```python
from build123d import *

# Parameters (mm, degrees)
SALIENTE_EXTRUIR1_DEPTH = 60
CORTAR_EXTRUIR1_DEPTH   = 10


with BuildPart() as part:
    # Croquis1 → Saliente-Extruir1 (new body)
    with BuildSketch(Plane.XY):
        with BuildLine():
            Line((-71.508108108, 44.822972973), (-71.508108108, 45.822972973))
            Line((-71.508108108, 45.822972973), (-21.508108108, 45.822972973))
            Line((-21.508108108, 45.822972973), (-21.508108108, 44.822972973))
            ThreePointArc((-21.508108108, 44.822972973), (-20.008108108, 43.322972973), (-21.508108108, 41.822972973))
            Line((-21.508108108, 41.822972973), (-21.508108108, 40.822972973))
            Line((-21.508108108, 40.822972973), (-71.508108108, 40.822972973))
            Line((-71.508108108, 40.822972973), (-71.508108108, 41.822972973))
            ThreePointArc((-71.508108108, 41.822972973), (-73.008108108, 43.322972973), (-71.508108108, 44.822972973))
        make_face()
    extrude(amount=SALIENTE_EXTRUIR1_DEPTH)

    # Croquis3 → Cortar-Extruir1 (cut)
    with BuildSketch(Plane(origin=(0, 0, 0), x_dir=(-1, 0, 0), z_dir=(0, 0, -1))):
        with BuildLine():
            Line((36.508108108, 41.322972973), (36.508108108, 40.822972973))
            Line((36.508108108, 40.822972973), (56.508108108, 40.822972973))
            Line((56.508108108, 40.822972973), (56.508108108, 41.322972973))
            ThreePointArc((56.508108108, 41.322972973), (55.92232167, 42.737186535), (54.508108108, 43.322972973))
            Line((54.508108108, 43.322972973), (38.508108108, 43.322972973))
            ThreePointArc((38.508108108, 43.322972973), (37.093894546, 42.737186535), (36.508108108, 41.322972973))
        make_face()
    extrude(amount=-CORTAR_EXTRUIR1_DEPTH, mode=Mode.SUBTRACT)


solid = part.part
```
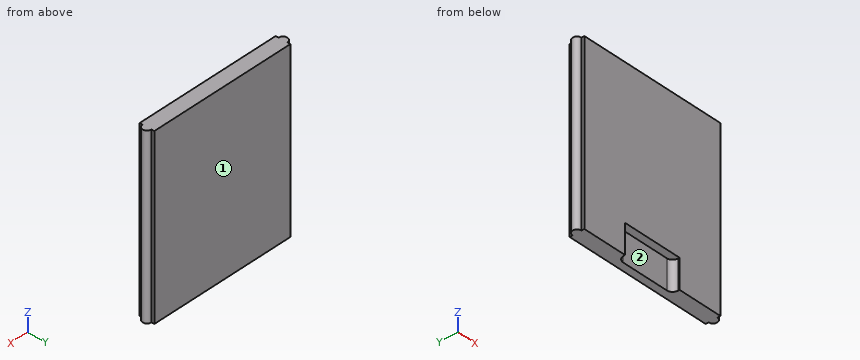
CAD build for the part. Positions are in the model's coordinates, mm. Face numbers are marked on the shaded views. Round coordinates to 2 decimals unless told otherwise and drop trailing zeros. Write each loop counter-clockwise with the first axis right and the second up, starting at its lowest first coordinate (ties: lowest second). Pieces come first, ordered by that corner, then holes.
Item 1: Mould opens along X. For the marked faces 1 and 2 say: released by +X, released by -X, zero draft, split by the parting line, or undercut.
Filled in:
face 1: zero draft
face 2: undercut
Item 2: Band-saw the part on A-A on z = 41. Write the cut outline in (x, y), then the cut area to 3 significant figures.
Filled in:
outline: (-71.51, 40.82) - (-21.51, 40.82) - (-21.51, 41.82) arc R1.5 ccw to (-21.51, 44.82) - (-21.51, 45.82) - (-71.51, 45.82) - (-71.51, 44.82) arc R1.5 ccw to (-71.51, 41.82) - close
area: 257 mm2
Item 3: Drop flat-ended pins along their axis: pin 1 Ø2 at (x, y) = (-46, 41.5) entering from -Z; pin 2 Ø0.5 at (y, z) = (45.5, 34) entering from -X; pin 3 Ø8 at (x, z) = (-46.5, 5.5) entering from -Y. Give the stop position or say it passes through.
Filled in:
pin 1: stops at z = 10
pin 2: stops at x = -71.51
pin 3: stops at y = 43.32
Item 4: Band-saw the part on B-B on x = -48.5. Write the cut outline in (y, z).
Filled in:
outline: (40.82, 10) - (43.32, 10) - (43.32, 0) - (45.82, 0) - (45.82, 60) - (40.82, 60) - close
Item 5: Drill centre lines: L1, parallel to X at y = 41.05, z = 5; L2, parallel to X at y = 41.7, z = 16.5; L3, parallel to Z at x = -51.5, y = 42.85. Where is each one in solid material? Low to high.
Filled in:
L1: x = -71.51 to -56.51, -36.51 to -21.51
L2: x = -71.51 to -21.51
L3: z = 10 to 60
Item 6: Band-saw the part on C-C on y = 42.65. Write the cut outline in (x, z), then the cut area to 3 significant figures.
Filled in:
outline: (-72.85, 0) - (-56, 0) - (-56, 10) - (-37.01, 10) - (-37.01, 0) - (-20.17, 0) - (-20.17, 60) - (-72.85, 60) - close
area: 2,970 mm2
